Here's the drawing with two shaded views (mm, measured from the low corner). I have some questions. Give positions to 0.01 mm unless a question says otherwise; leave off trailing zeros. Write each loop counter-clockwise with the first axis right and the second up, starting at its lowest first coordinate (ties: lowest second). Pieces come first, ordered by that corner, then holes. Notation, with made-up numbers: (21.25, 11.5) -> (77.25, 11.5) arc R19 ccw to (77.25, 39.5) -> close; hole circle Ø1 at (24, 68). An arc over 180 degrees is marked (long way). One line per item, written item: value.
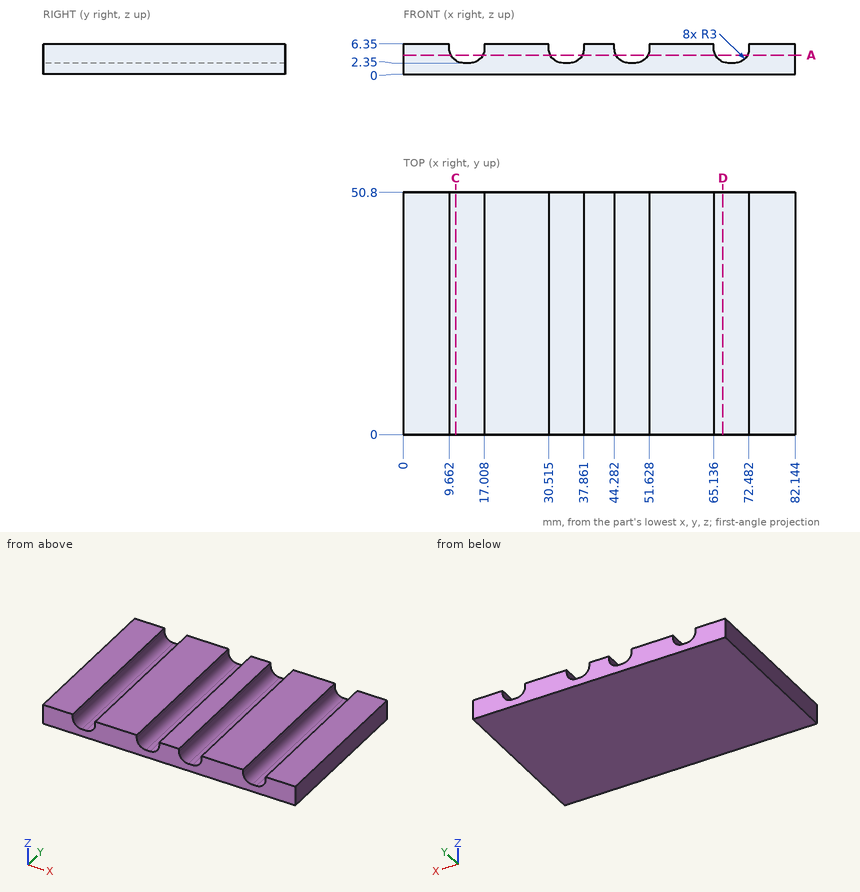
1) If we section it at A-A (z = 4): Write out the boundary of the cut face in (x, y).
Answer list:
outline: (0, 0) -> (9.98, 0) -> (9.98, 50.8) -> (0, 50.8) -> close; (16.69, 0) -> (30.84, 0) -> (30.84, 50.8) -> (16.69, 50.8) -> close; (37.54, 0) -> (44.6, 0) -> (44.6, 50.8) -> (37.54, 50.8) -> close; (51.31, 0) -> (65.46, 0) -> (65.46, 50.8) -> (51.31, 50.8) -> close; (72.16, 0) -> (82.14, 0) -> (82.14, 50.8) -> (72.16, 50.8) -> close
2) I need wall thicknesses on L1, parallel to X at y = 13.5, z = 5.75 (1 decimal); L2, parallel to X at y = 4, z = 2.75 (1 decimal); L3, parallel to Z at x = 47.5, y = 18.5. Which ranges of each line are inside material? Lowest first, please.
Answer list:
L1: x = 0 to 9.7, 17 to 30.5, 37.9 to 44.3, 51.6 to 65.1, 72.5 to 82.1
L2: x = 0 to 11.2, 15.5 to 32, 36.4 to 45.8, 50.1 to 66.6, 71 to 82.1
L3: z = 0 to 2.35
3) Will these pins go through, and if not, where does the flat tip stop? pin 1 (1.5 mm diameter, centred on x = 69, y = 22, fed in from +Z); pin 2 (0.7 mm diameter, centred on x = 48, y = 15, fed in from +Z).
Answer list:
pin 1: stops at z = 2.36
pin 2: stops at z = 2.35
4) If we section it at D-D (x = 67): Write out the boundary of the cut face in (y, z), and give its area (3 significant figures).
Answer list:
outline: (0, 0) -> (50.8, 0) -> (50.8, 2.57) -> (0, 2.57) -> close
area: 131 mm^2
5) If we section it at C-C (x = 11): Write out the boundary of the cut face in (y, z), and give its area (3 significant figures).
Answer list:
outline: (0, 0) -> (50.8, 0) -> (50.8, 2.85) -> (0, 2.85) -> close
area: 145 mm^2
